Part print with two shaded views. Sizes in mm from the minimum x, y, z corner. A direction names the side the tool comes from. Give positions to 0.01 mm unless a question says otherwise; leave off trailing zeros. Order: outer loops, then holes, each group sorted by start corner. A loop starts at its lowest first (then second) coordinate and runs counter-clockwise, first axis right, second up. Notation, with made-up numbers: M 81,43.5 L 99,43.5 A16 cw 99,71.5 Z; hole C -3,31.25 d3. An arc over 180 degrees is marked long. Answer as CSV lines item,"result".
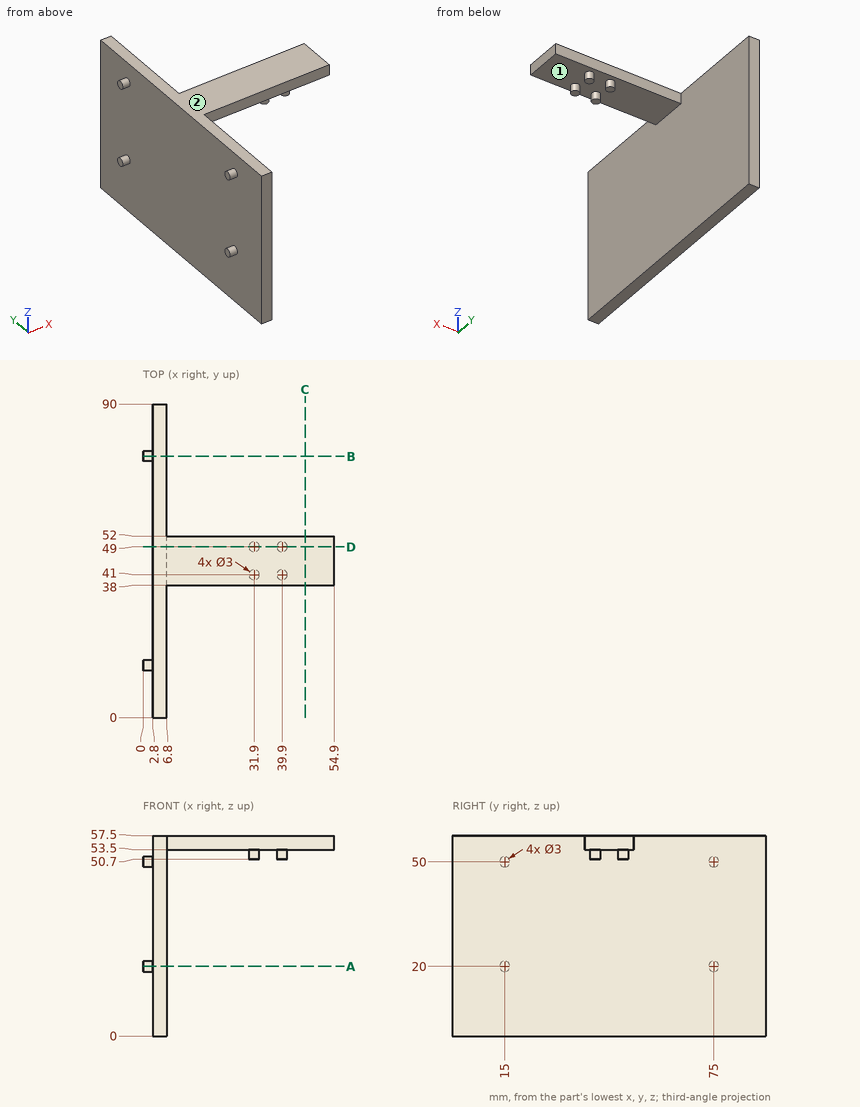
Item 1: Drop flat-ended pins along their axis: pin 1 (1.5 mm diameter, centred on x = 39.5, y = 40.5, fed in from -Z); pin 2 (3 mm diameter, centred on y = 25.5, z = 33, fed in from -X); pin 3 (3 mm diameter, centred on x = 42.5, z = 55, fed in from -Y). Give the stop position or say it passes through.
Geometry says:
pin 1,"stops at z = 50.7"
pin 2,"stops at x = 2.8"
pin 3,"stops at y = 38"
Item 2: Band-saw the part on D-D (y = 49). Give the cut face in (x, z).
Geometry says:
outline,"M 2.8,0 L 6.8,0 L 6.8,53.5 L 30.4,53.5 L 30.4,50.7 L 33.4,50.7 L 33.4,53.5 L 38.4,53.5 L 38.4,50.7 L 41.4,50.7 L 41.4,53.5 L 54.9,53.5 L 54.9,57.5 L 2.8,57.5 Z"
Item 3: 3-axis set-ups, long thin cutter, end or side, ignore diameter. For the marked faces 1 and 2: which of +Z, -Z, +X, -X, +Y, -Y reach the whole face in a straight line?
Geometry says:
face 1,"-Z"
face 2,"+Z, +X, -X, +Y, -Y"
Item 4: Band-saw the part on A-A (z = 20). Give the cut face in (x, y), and give its area (3 significant figures).
Geometry says:
outline,"M 0,13.5 L 2.8,13.5 L 2.8,0 L 6.8,0 L 6.8,90 L 2.8,90 L 2.8,76.5 L 0,76.5 L 0,73.5 L 2.8,73.5 L 2.8,16.5 L 0,16.5 Z"
area,"377 mm2"
Item 5: Probe line 1 along X through (y, z) = (16, 45.5); line 2 along Z through (x, y) = (42.5, 46); line 3 along Y through (x, z) = (39, 53). List the from-to ranges inside material, lowest first. Write a range as from..to.
Geometry says:
line 1,"x = 2.8..6.8"
line 2,"z = 53.5..57.5"
line 3,"y = 39.8..42.2, 47.8..50.2"
Item 6: Band-saw the part on B-B (y = 75). Give the cut face in (x, z).
Geometry says:
outline,"M 0,18.5 L 2.8,18.5 L 2.8,0 L 6.8,0 L 6.8,57.5 L 2.8,57.5 L 2.8,51.5 L 0,51.5 L 0,48.5 L 2.8,48.5 L 2.8,21.5 L 0,21.5 Z"
Item 7: Band-saw the part on C-C (x = 46.5). Give the cut face in (y, z).
Geometry says:
outline,"M 38,53.5 L 52,53.5 L 52,57.5 L 38,57.5 Z"
